Autodesk Inventor part; units mm, degrees
ref_plane "YZ Plane" through (0, 0, 0) normal (1, 0, 0) x (0, 1, 0)
ref_plane "XZ Plane" through (0, 0, 0) normal (0, 1, 0) x (-1, 0, 0)
ref_plane "XY Plane" through (0, 0, 0) normal (0, 0, 1) x (1, 0, 0)
ref_plane "Płaszczyzna konstrukcyjna1" through (0, 0, 0) normal (0, 0, 1) x (1, 0, 0)
sketch "Szkic1" plane through (0, 0, 0) normal (0, 0, 1) x (1, 0, 0)
  circle A0 centre (836, 698.5) radius 4
  circle A1 centre (836, 98.5) radius 4
  circle A2 centre (698.5, -39) radius 4
  circle A3 centre (98.5, -39) radius 4
  circle A4 centre (-39, 98.5) radius 4
  circle A5 centre (-39, 698.5) radius 4
  circle A6 centre (836, 398.5) radius 4
  circle A7 centre (398.5, -39) radius 4
  circle A8 centre (-39, 398.5) radius 4
  circle A9 centre (98.5, 836) radius 4
  circle A10 centre (698.5, 836) radius 4
  circle A11 centre (398.5, 836) radius 4
  line L0 (0, 797) -> (0, 0)
  line L1 (0, 0) -> (797, 0)
  line L2 (797, 0) -> (797, 797)
  line L3 (797, 797) -> (0, 797)
  line L4 (856, 856) -> (856, -59)
  line L5 (856, -59) -> (-59, -59)
  line L6 (-59, -59) -> (-59, 856)
  line L7 (-59, 856) -> (856, 856)
  line L8 (406, 797) -> (391, 797)
  line L9 (391, 797) -> (391, 0)
  line L10 (391, 0) -> (406, 0)
  line L11 (406, 0) -> (406, 797)
  line L12 (406, 797) -> (391, 0) construction
  line L13 (391, 797) -> (406, 0) construction
  line L14 (797, 406) -> (0, 406)
  line L15 (0, 406) -> (0, 391)
  line L16 (0, 391) -> (797, 391)
  line L17 (797, 391) -> (797, 406)
  line L18 (797, 406) -> (0, 391) construction
  line L19 (0, 406) -> (797, 391) construction
  circle A12 centre (761, -24) radius 3
  circle A13 centre (348.5, -24) radius 3
  circle A14 centre (-24, -24) radius 3
  circle A15 centre (-24, 348.5) radius 3
  circle A16 centre (-24, 761) radius 3
  circle A17 centre (248.5, 821) radius 3
  circle A18 centre (648.5, 821) radius 3
  circle A19 centre (821, 648.5) radius 3
  circle A20 centre (821, 248.5) radius 3
  circle A21 centre (821, 348.5) radius 3
  circle A22 centre (821, 761) radius 3
  circle A23 centre (548.5, 821) radius 3
  circle A24 centre (148.5, 821) radius 3
  circle A25 centre (-24, 648.5) radius 3
  circle A26 centre (-24, 248.5) radius 3
  circle A27 centre (36, -24) radius 3
  circle A28 centre (448.5, -24) radius 3
  circle A29 centre (821, -24) radius 3
  circle A30 centre (648.5, -24) radius 3
  circle A31 centre (248.5, -24) radius 3
  circle A32 centre (-24, 36) radius 3
  circle A33 centre (-24, 448.5) radius 3
  circle A34 centre (-24, 821) radius 3
  circle A35 centre (348.5, 821) radius 3
  circle A36 centre (761, 821) radius 3
  circle A37 centre (821, 548.5) radius 3
  circle A38 centre (821, 148.5) radius 3
  circle A39 centre (821, 448.5) radius 3
  circle A40 centre (821, 821) radius 3
  circle A41 centre (448.5, 821) radius 3
  circle A42 centre (36, 821) radius 3
  circle A43 centre (-24, 548.5) radius 3
  circle A44 centre (-24, 148.5) radius 3
  circle A45 centre (148.5, -24) radius 3
  circle A46 centre (548.5, -24) radius 3
  circle A47 centre (821, 36) radius 3
  point P0 (398.5, 398.5)
  point P1 (391, 391)
  point P2 (406, 391)
  point P3 (797, 391)
  point P4 (797, 406)
  point P5 (406, 406)
  point P6 (391, 406)
  point P7 (0, 406)
  dimension "d6" = 15
  dimension "d7" = 797
  dimension "d8" = 15
extrude "Wyciągnięcie proste1" add sketch "Szkic1" along normal blind 3 contours L14 L9 L16 L0 | L3 L11 L14 L9 | L14 L11 L16 L9 | L16 L11 L1 L9 | L14 L2 L16 L11
properties part number "krys" material "Aluminium"
Geometry: final body of the model. Coordinates: model frame, mm. Round coordinates to 2 decimals unless told otherwise and drop trailing zeros. Write each loop counter-clockwise with the first axis right and the second up, starting at its lowest first coordinate (ties: lowest second). Pieces come first, ordered by that corner, then holes.
Item 1: Section query B-B (y = 636). Return loops of the section in (x, z), plus the area to 3 significant figures.
Item 2: Material intervals for L1, parallel to Y at x = 152, z = 2.1, sorted ascending.
Item 3: Pin query (flat end, axial travel): P1, Ø1.5, axis at y = 115.5, z = 2, coming from the +X side; P2, Ø1, axis at x = 314, z = 1, coming from the +Y side; P3, Ø1.5, axis at x = 166, z = 1.5, coming from the -Y side. Return the tip coordinate at first contact, or that it passes through.
Item 4: Section query A-A (z = 0.65). Return loops of the section in (x, y).
Completed:
1. outline: (391, 0) - (406, 0) - (406, 3) - (391, 3) - close
1. area: 45.0 mm2
2. L1: y = 391 to 406
3. P1: stops at x = 406
3. P2: stops at y = 406
3. P3: stops at y = 391
4. outline: (0, 391) - (391, 391) - (391, 0) - (406, 0) - (406, 391) - (797, 391) - (797, 406) - (406, 406) - (406, 797) - (391, 797) - (391, 406) - (0, 406) - close
